```python
from build123d import *

# Parameters (mm, degrees)
F0_W      = 114.278237
F0_H      = 55
F1_DEPTH  = 30
F2_W      = 43.190174
F2_H      = 32.801846
F3_DEPTH  = 30.001
F4_W      = 7.815801
F4_H      = 9.223189
F5_DEPTH  = 3
F6_W      = 4.690871
F6_H      = 6.195421
F7_DEPTH  = 7
F8_W      = 16.93508
F8_H      = 10.262838
F9_DEPTH  = 5
F10_R     = 3.555014
F11_DEPTH = 8
F12_R     = 6.524901
F13_DEPTH = 5
F14_R     = 2.620041
F15_DEPTH = 10


with BuildPart() as f1:
    # F0 (on Top) → F1 (new body)
    with BuildSketch(Plane.XY):
        with Locations((-57.139118, 27.5)):
            Rectangle(F0_W, F0_H)
    extrude(amount=F1_DEPTH)

    # F2 (on face) → F3 (cut, through all)
    with BuildSketch(Plane.XY.offset(30)):
        with Locations((-78.348886, 28.64116)):
            Rectangle(F2_W, F2_H)
    extrude(amount=-F3_DEPTH, mode=Mode.SUBTRACT)

    # F4 (on face) → F5 (join)
    with BuildSketch(Plane(origin=(0, 12.240237, 0), x_dir=(-1, 0, 0), z_dir=(0, 1, 0))):
        with Locations((89.257304, 9.994802)):
            Rectangle(F4_W, F4_H)
    extrude(amount=F5_DEPTH)

    # F6 (on face) → F7 (join)
    with BuildSketch(Plane(origin=(0, 12.240237, 0), x_dir=(-1, 0, 0), z_dir=(0, 1, 0))):
        with Locations((74.541517, 22.166014)):
            Rectangle(F6_W, F6_H)
    extrude(amount=F7_DEPTH)

    # F8 (on face) → F9 (join)
    with BuildSketch(Plane(origin=(0, 12.240237, 0), x_dir=(-1, 0, 0), z_dir=(0, 1, 0))):
        with Locations((69.395147, 9.889492)):
            Rectangle(F8_W, F8_H)
    extrude(amount=F9_DEPTH)

    # F10 (on face) → F11 (join)
    with BuildSketch(Plane.XZ.offset(-45.042083)):
        with Locations((-92.950813, 12.721915)):
            Circle(F10_R)
    extrude(amount=F11_DEPTH)

    # F12 (on face) → F13 (join)
    with BuildSketch(Plane.XZ.offset(-45.042083)):
        with Locations((-81.588104, 18.474752)):
            Circle(F12_R)
    extrude(amount=F13_DEPTH)

    # F14 (on face) → F15 (join)
    with BuildSketch(Plane.XZ.offset(-45.042083)):
        with Locations((-67.019306, 5.002084)):
            Circle(F14_R)
    extrude(amount=F15_DEPTH)


solid = f1.part
```
Input: part model. Units: mm. Frame: model coordinates. A direction names the side the tool comes from. Round coordinates to 2 decimals unless told otherwise and drop trailing zeros. Loops run counter-clockwise (first coordinate to the right, second up) from the corner with the lowest first, then second, coordinate; pieces in that order, holes last. Notation, with made-up numbers: (-14.75, 2.5) -> (2.25, 2.5) arc R10 cw to (2.25, 9.5) -> close; hole circle Ø7 at (62.25, -11.75). An arc over 180 degrees is marked (long way). Use one line per item in the form item = value. Start each with the question number.
Item 1: Material intervals for L1, parallel to X at y = 14.5, z = 9.75; L2, parallel to Y at x = -88.5, z = 13.75; L3, parallel to X at y = 22.5, z = 13.25, sorted ascending. Write a range as from..to.
Item 2: Contact query for flat-ended pins moving along their axis: pin 1 Ø3.5 at (x, y) = (-90, 14.5) entering from -Z; pin 2 Ø4 at (x, y) = (-74.5, 15.5) entering from -Z; pin 3 Ø1.5 at (x, y) = (-90, 14) entering from +Z. Output: stop coordinate, or through.
Item 3: Section query D-D on z = 20.25. Return the cut outline in (x, y), then the cut area to 3 significant figures.
Item 4: Mould query, pull axis Y, two halves, no side actions, for faces 1 (the face through (0, 27, 15)), 2 (the face through (-58, 0, 15)), 3 (the face through (-82, 40.042, 19)). Classes: pulls with the +Y half, pulls with the -Y half, needs draft (parallel to the pull), parting line crosses it, or undercut.
Item 5: Section query C-C on x = -84. Return the cut outline in (y, z).
Item 6: Section query A-A on y = 20.5. Return the cut outline in (x, z), then the cut area to 3 significant figures.
Item 7: Section query B-B on z = 26.75. Return the cut outline in (x, y), then the cut area to 3 significant figures.
Item 8: Set-up query: faces 4 (the face through (-60.928, 15, 10)), 5 (the face through (-69, 17.24, 10)), 6 (the face through (-88.107, 42.577, 18.762)). Return all of +Z, -Z, +X, -X, +Y, -Y with unobstructed straight access to the full face (end or side cutting, diameter ignored); none if empty.
Ans:
q1.L1 = -114.28..-99.94, -93.17..-85.35, -77.86..-60.93, -56.75..0
q1.L2 = 0..15.24, 45.04..55
q1.L3 = -114.28..-99.94, -56.75..0
q2.pin_1 = 5.38
q2.pin_2 = 4.76
q2.pin_3 = 14.61
q3.outline = (-114.28, 0) -> (0, 0) -> (0, 55) -> (-114.28, 55) -> close; hole (-99.94, 12.24) -> (-76.89, 12.24) -> (-76.89, 19.24) -> (-72.2, 19.24) -> (-72.2, 12.24) -> (-56.75, 12.24) -> (-56.75, 45.04) -> (-75.31, 45.04) -> (-75.31, 40.04) -> (-87.87, 40.04) -> (-87.87, 45.04) -> (-99.94, 45.04) -> close
q3.area = 4,960 mm^2
q4.face_1 = needs draft
q4.face_2 = pulls with the -Y half
q4.face_3 = undercut
q5.outline = (0, 0) -> (12.24, 0) -> (12.24, 30) -> (0, 30) -> close; (40.04, 12.41) -> (45.04, 12.41) -> (45.04, 0) -> (55, 0) -> (55, 30) -> (45.04, 30) -> (45.04, 24.54) -> (40.04, 24.54) -> close
q6.outline = (-114.28, 0) -> (-99.94, 0) -> (-99.94, 30) -> (-114.28, 30) -> close; (-56.75, 0) -> (0, 0) -> (0, 30) -> (-56.75, 30) -> close
q6.area = 2,130 mm^2
q7.outline = (-114.28, 0) -> (0, 0) -> (0, 55) -> (-114.28, 55) -> close; hole (-99.94, 12.24) -> (-56.75, 12.24) -> (-56.75, 45.04) -> (-99.94, 45.04) -> close
q7.area = 4,870 mm^2
q8.face_4 = +Z, -Z
q8.face_5 = -Z
q8.face_6 = none
